from build123d import *

# Parameters (mm, degrees)
SKETCH1_W           = 24
SKETCH1_H           = 24
SKETCH1_R           = 2
BOSS_EXTRUDE1_DEPTH = 2
SKETCH1_3_W         = 24
SKETCH1_3_H         = 2
BOSS_EXTRUDE2_DEPTH = 26
SKETCH2_R           = 2
CUT_EXTRUDE1_DEPTH  = 26


with BuildPart() as part:
    # Sketch1 → Boss-Extrude1 (new body)
    with BuildSketch(Plane(origin=(0, 0, 0), x_dir=(1, 0, 0), z_dir=(0, 1, 0))):
        with Locations((0, -1)):
            Rectangle(SKETCH1_W, SKETCH1_H)
        with Locations(Location((-8, -8, 0), (0, 0, 270))):
            Circle(SKETCH1_R, mode=Mode.SUBTRACT)
        with Locations(Location((-8, 0, 0), (0, 0, 270))):
            Circle(SKETCH1_R, mode=Mode.SUBTRACT)
        with Locations(Location((0, -8, 0), (0, 0, 270))):
            Circle(SKETCH1_R, mode=Mode.SUBTRACT)
        with Locations(Location((8, -8, 0), (0, 0, 270))):
            Circle(SKETCH1_R, mode=Mode.SUBTRACT)
        with Locations(Location((0, 0, 0), (0, 0, 270))):
            Circle(SKETCH1_R, mode=Mode.SUBTRACT)
        with Locations(Location((8, 0, 0), (0, 0, 270))):
            Circle(SKETCH1_R, mode=Mode.SUBTRACT)
        with Locations(Location((-8, 8, 0), (0, 0, 270))):
            Circle(SKETCH1_R, mode=Mode.SUBTRACT)
        with Locations(Location((0, 8, 0), (0, 0, 270))):
            Circle(SKETCH1_R, mode=Mode.SUBTRACT)
        with Locations(Location((8, 8, 0), (0, 0, 270))):
            Circle(SKETCH1_R, mode=Mode.SUBTRACT)
    extrude(amount=BOSS_EXTRUDE1_DEPTH)

    # Sketch1_3 → Boss-Extrude2 (add)
    with BuildSketch(Plane(origin=(0, 0, 0), x_dir=(1, 0, 0), z_dir=(0, 1, 0))):
        with Locations((0, 12)):
            Rectangle(SKETCH1_3_W, SKETCH1_3_H)
    extrude(amount=BOSS_EXTRUDE2_DEPTH)

    # Sketch2 → Cut-Extrude1 (cut)
    with BuildSketch(Plane.XY.offset(-11)):
        with Locations((-8, 22)):
            Circle(SKETCH2_R)
        with Locations((0, 22)):
            Circle(SKETCH2_R)
        with Locations((8, 22)):
            Circle(SKETCH2_R)
        with Locations((-8, 14)):
            Circle(SKETCH2_R)
        with Locations((0, 14)):
            Circle(SKETCH2_R)
        with Locations((8, 14)):
            Circle(SKETCH2_R)
        with Locations((8, 6)):
            Circle(SKETCH2_R)
        with Locations((0, 6)):
            Circle(SKETCH2_R)
        with Locations((-8, 6)):
            Circle(SKETCH2_R)
    extrude(amount=-CUT_EXTRUDE1_DEPTH, mode=Mode.SUBTRACT)


solid = part.part
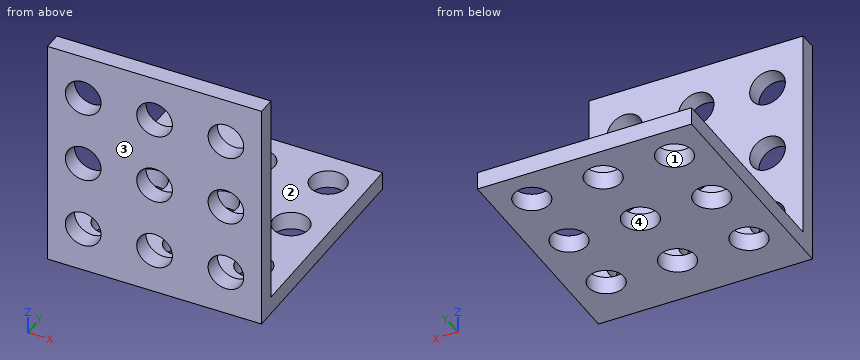
Work out the finished part from the listing and answer in its coordinate system (mm). Face numbers are marked on the shaded views. A direction names the side the tool comes from. Give positions to 0.01 mm unless a question says otherwise; leave off trailing zeros. Loops run counter-clockwise (first coordinate to the right, second up) from the corner with the lowest first, then second, coordinate; pieces in that order, holes last. Notation, with made-up numbers: (72.5, -39.5) - (129.5, -39.5) arc R27 cw to (129.5, -9.5) - close; hole circle Ø4 at (67, -13). An arc over 180 degrees is marked (long way). Answer in a Markdown table with one row per item. Add a question column.
Q1. The part is cut by section D-D (y = 10.75). Determine the outline of the cut face in (x, z), and give its area (3 significant figures).
Q2. The part is cut by section C-C (x = -8). State how many separate pieces and enclosed holes the cut face has, and give its area (3 significant figures).
Q3. Consider line 1 along X through (y, z) = (0.9, 8); line 2 along Y through (x, z) = (-8, -11.65); line 3 along Y through (x, z) = (-5, -2). Determine where each line is inside the solid, lowest interval first.
Q4. A tool of negligible diameter and unlimited length cuts with its end or side. For the marked faces 1 and 2, from which of +Z, -Z, +X, -X, +Y, -Y can it reach the whole face along a straight path? Write none if from no direction.
Q5. The part is cut by section A-A (z = -8). Determine the outline of the cut face in (x, y), and give its area (3 significant figures).
Q6. Determine the mould class of the marked faces 3 and 4 for opening direction X: released by +X, released by -X, zero draft, split by the parting line, or undercut.
Q7. The part is cut by section B-B (y = 22). Determine the outline of the cut face in (x, z), and give its area (3 significant figures).
Q8. Each of these flat-tipped pins is pushed along its axis until it touches: P1, Ø12, axis at x = -2.5, z = -4, coming from the +Y side; P2, Ø12, axis at x = 1, y = 17, coming from the +Z side; P3, Ø2.5, axis at x = 8, y = 6, coming from the -Z side. Where does it stop, or does it pass through?
Solution:
| question | item | result |
|---|---|---|
| 1 | outline | (-12, -13) - (12, -13) - (12, -11) - (-12, -11) - close |
| 1 | area | 48.0 mm² |
| 2 | separate pieces | 7 |
| 2 | enclosed holes | 0 |
| 2 | area | 52.0 mm² |
| 3 | line 1 | x = -12 to -10, -6 to -2, 2 to 6, 10 to 12 |
| 3 | line 2 | y = 0 to 4, 8 to 12, 16 to 20, 24 to 26 |
| 3 | line 3 | y = 0 to 2 |
| 4 | face 1 | +Z, -Z |
| 4 | face 2 | +Z, +X, -X, +Y |
| 5 | outline | (-12, 0) - (-10, 0) - (-10, 2) - (-12, 2) - close; (-6, 0) - (-2, 0) - (-2, 2) - (-6, 2) - close; (2, 0) - (6, 0) - (6, 2) - (2, 2) - close; (10, 0) - (12, 0) - (12, 2) - (10, 2) - close |
| 5 | area | 24.0 mm² |
| 6 | face 3 | zero draft |
| 6 | face 4 | undercut |
| 7 | outline | (-12, -13) - (-10, -13) - (-10, -11) - (-12, -11) - close; (-6, -13) - (-2, -13) - (-2, -11) - (-6, -11) - close; (2, -13) - (6, -13) - (6, -11) - (2, -11) - close; (10, -13) - (12, -13) - (12, -11) - (10, -11) - close |
| 7 | area | 24.0 mm² |
| 8 | P1 | stops at y = 2 |
| 8 | P2 | stops at z = -11 |
| 8 | P3 | passes through |
